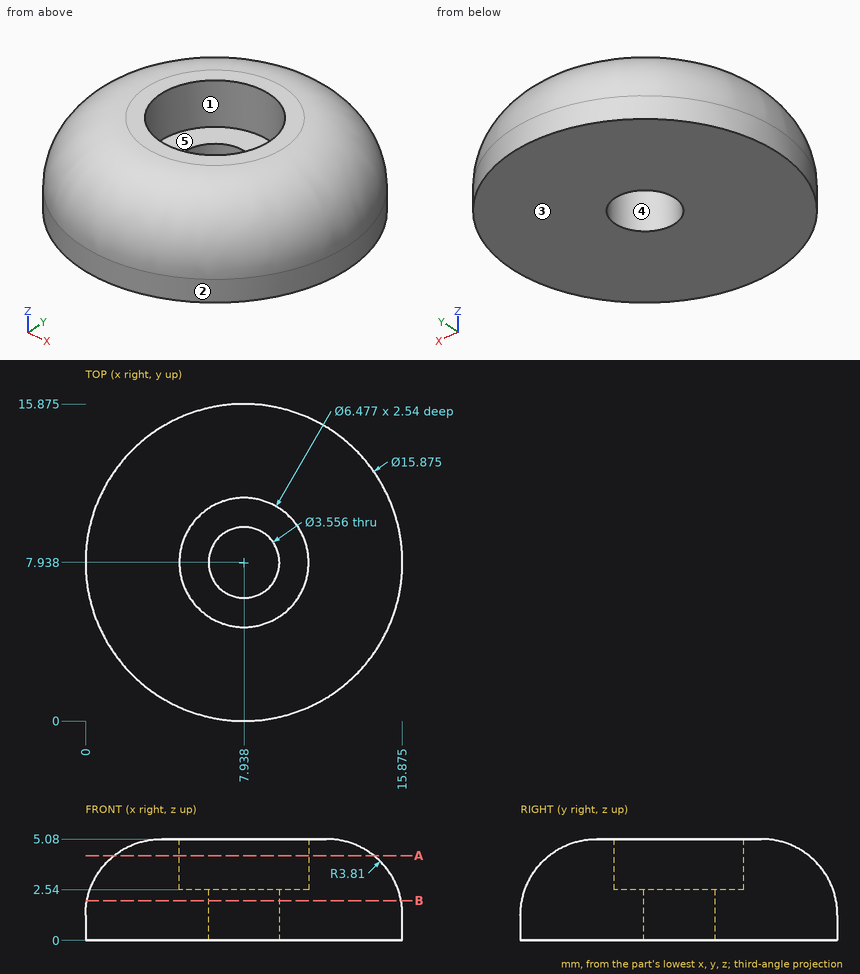
Verification items for this drawing (mm, ordinates from the low corner). A direction names the side the tool comes from. Coordinates: 2 decimals unless noted, no trailing zeros. Order: outer loops, then holes, each group sorted by start corner. A loop starts at its lowest first (then second) coordinate and runs counter-clockwise, first axis right, second up. Notation, with made-up numbers: (41.5, 88) - (73.5, 88) arc R18 ccw to (73.5, 108) - close; hole circle Ø6 at (53, 82). An arc over 180 degrees is marked (long way). Answer in a Markdown table with one row per item. Add a question column.
1. Gauge pin test, flat ends, axial feed: pin 1 Ø1 at (x, z) = (13, 4) entering from -Y (1 decimal); pin 2 Ø3 at (y, z) = (12, 1) entering from -X (1 decimal); pin 3 Ø5.5 at (x, y) = (7.94, 7.94) entering from -Z; pin 4 Ø1 at (x, z) = (7.5, 3.5) entering from -Y. Record the tip position at first contact, or that the pin passes through.
2. Access from +Z, -Z, +X, -X, +Y, -Y to the whole of each face (thin tool, end or side, straight path). Record for the marked faces 4 and 5.
3. Draft check along X on the marked faces 1, 2 and 3. Enter one of: +X half, -X half, draft (parallel to the pull), parting line (faces both ways), or undercut.
4. Material ranges on L1, parallel to Z at x = 8.25, y = 12.25 (1 decimal); L2, parallel to Z at x = 9.75, y = 5.75; L3, parallel to X at y = 10, z = 3 (1 decimal), recorded low to high. Write a range as [from, to].
5. Section check B-B (z = 2). Enter the section's corners in (x, y) (1 decimal).
6. Section check A-A (z = 4.25). Enter the section's corners in (x, y) (1 decimal).
Data:
| question | item | result |
|---|---|---|
| 1 | pin 1 | stops at y = 2.6 |
| 1 | pin 2 | stops at x = 0.4 |
| 1 | pin 3 | stops at z = 0 |
| 1 | pin 4 | stops at y = 0.43 |
| 2 | face 4 | +Z, -Z |
| 2 | face 5 | +Z |
| 3 | face 1 | undercut |
| 3 | face 2 | parting line |
| 3 | face 3 | draft |
| 4 | L1 | z = [0, 5.1] |
| 4 | L2 | z = [0, 2.54] |
| 4 | L3 | x = [0.7, 5.4], [10.4, 15.2] |
| 5 | outline | circle Ø15.7 at (7.9, 7.9); hole circle Ø3.6 at (7.9, 7.9) |
| 6 | outline | circle Ø13 at (7.9, 7.9); hole circle Ø6.5 at (7.9, 7.9) |
